from build123d import *

# Parameters (mm, degrees)
F0_W        = 65
F0_H        = 37
F1_DEPTH    = 25
F2_R        = 5
F3_T1_DEPTH = 32.5
F3_S5_W     = 5
F3_S5_H     = 5
F3_T6_DEPTH = 5


# Not quite as in the source:
# - a fillet or chamfer that OpenCascade refuses, or shapes differently, is made with other operations: its cross-section is extruded or revolved along the edge and cut away or added


with BuildPart() as f1:
    # F0 (on Front) → F1 (new body)
    with BuildSketch(Plane.XZ):
        Rectangle(F0_W, F0_H)
    extrude(amount=F1_DEPTH)

    # F2
    f2_edges = [f1.edges().sort_by_distance(p)[0] for p in [
        (-32.5, -12.5, 18.5),
        (-32.5, -12.5, -18.5),
        (0, 0, 18.5),
        (-32.5, 0, 0),
        (32.5, 0, 0),
        (32.5, -12.5, -18.5),
        (0, 0, -18.5),
    ]]
    fillet(f2_edges, radius=F2_R)

    # F3: fillet of radius 5 on 1 edges, made by hand

    # F3_s2 → F3_t1 (cut)
    with BuildSketch(Plane.XZ.offset(5)):
        with BuildLine():
            ThreePointArc((27.5, 18.5), (31.0355339059, 17.0355339059), (32.5, 13.5))
            Line((32.5, 13.5), (32.5, 18.5))
            Line((32.5, 18.5), (27.5, 18.5))
        make_face()
    extrude(amount=F3_T1_DEPTH, mode=Mode.SUBTRACT)


with BuildPart() as f3_tool4:
    # F3_s5 → F3_t6 (new body)
    with BuildSketch(Plane.XY.offset(13.5)):
        with Locations((30, -2.5)):
            Rectangle(F3_S5_W, F3_S5_H)
    extrude(amount=F3_T6_DEPTH)

    # F3_s7 → F3_t8 (revolve, cut)
    with BuildSketch(Plane(origin=(27.5, -5, 13.5), x_dir=(-0.7071067812, -0.7071067812, 0), z_dir=(-0.7071067812, 0.7071067812, 0))):
        with BuildLine():
            ThreePointArc((0, -5), (5, 0), (0, 5))
            Line((0, 5), (0, -5))
        make_face()
    revolve(axis=Axis((27.5, -5, 13.5), (0, 0, 1)), mode=Mode.SUBTRACT)


with BuildPart() as f1_1:
    add(f1.part)

    # F3_t3: cut F3_tool4
    add(f3_tool4.part, mode=Mode.SUBTRACT)


solid = f1_1.part
Work out the finished part from the listing and answer in its coordinate system (mm). Give positions to 0.01 mm unless a question says otherwise; leave off trailing zeros. Loops run counter-clockwise (first coordinate to the right, second up) from the corner with the lowest first, then second, coordinate; pieces in that order, holes last. Notation, with made-up numbers: (-28, 56.25) -> (26, 56.25) arc R20 ccw to (26, 92.25) -> close; hole circle Ø11 at (80.25, 54). An arc over 180 degrees is marked (long way). Use a Markdown table: item, result. Add a question column.
1. Section B-B on z = -16 is taken. Determine the outline of the cut face in (x, y).
2. A flat-ended cylindrical pin translates along its axis: pin 1 Ø1 at (y, z) = (-9.5, 15) entering from -X. Find the tip coordinate at first contact, or state that the pin passes through.
3. Find the intervals of material crossed by probe 1 along Z at (x, y) = (-30, -10.75); probe 2 along X at (y, z) = (-17, -16); probe 3 along X at (y, z) = (-20, 14), in increasing order.
4. Section A-A on z = 15 is taken. Determine the outline of the cut face in (x, y), and give its area (3 significant figures).
Results below:
| question | item | result |
|---|---|---|
| 1 | outline | (-31.83, -25) -> (31.83, -25) -> (31.83, -5) arc R4.33 ccw to (27.5, -0.67) -> (-27.5, -0.67) arc R4.33 ccw to (-31.83, -5) -> close |
| 2 | pin 1 | stops at x = -32.4 |
| 3 | probe 1 | z = -17.83 to 17.83 |
| 3 | probe 2 | x = -31.83 to 31.83 |
| 3 | probe 3 | x = -32.47 to 32.47 |
| 4 | outline | (-32.27, -25) -> (32.27, -25) -> (32.27, -5) arc R4.77 ccw to (27.5, -0.23) -> (-27.5, -0.23) arc R4.77 ccw to (-32.27, -5) -> close |
| 4 | area | 1,590 mm^2 |
